from build123d import *

# Parameters (mm, degrees)
F0_R     = 45
F0_R_2   = 3
F1_DEPTH = 25
F2_COUNT = 7


# Not quite as in the source:
# - a feature names something its author has since deleted; it is built from what else it names


with BuildPart() as f1:
    # F0 (on Front) → F1 (new body)
    with BuildSketch(Plane.XZ):
        Circle(F0_R)
        with BuildLine():
            ThreePointArc((40, 0), (-34.8753984239, -19.58842987), (20.8146707615, 34.1577148107))
            ThreePointArc((20.8146707615, 34.1577148107), (21.2557560399, 33.8849942478), (21.693268588, 33.6065781949))
            ThreePointArc((21.693268588, 33.6065781949), (35.126419854, 19.1346447116), (40, 0))
        make_face(mode=Mode.SUBTRACT)
        with BuildLine():
            ThreePointArc((20.8146707615, 34.1577148107), (4.7404997755, 21.9880977011), (-2.457993575, 3.1556722874))
            ThreePointArc((-2.457993575, 3.1556722874), (-0.7771850997, -3.9237715684), (3.4753115022, 1.9804570085))
            ThreePointArc((3.4753115022, 1.9804570085), (8.7719800119, 19.9895662469), (21.693268588, 33.6065781949))
            ThreePointArc((21.693268588, 33.6065781949), (21.2557560399, 33.8849942478), (20.8146707615, 34.1577148107))
        make_face()
        Circle(F0_R_2, mode=Mode.SUBTRACT)
    extrude(amount=F1_DEPTH)

    # F2: F1 ×7 about axis
    f2_axis = Axis((0, -25, 0), (0, -1, 0))


with BuildPart() as f1_1:
    add(f1.part)
    for i in range(1, F2_COUNT):
        add(f1.part.rotate(f2_axis, i * 360 / F2_COUNT))


solid = f1_1.part
Model file for the job. Use its own axes, mm. Give positions to 0.01 mm unless a question says otherwise; leave off trailing zeros. Order: outer loops, then holes, each group sorted by start corner. A loop starts at its lowest first (then second) coordinate and runs counter-clockwise, first axis right, second up. Notation, with made-up numbers: (-31.5, -8.5) - (19.5, -8.5) arc R19 cw to (19.5, 6.5) - close; hole circle Ø1 at (-32.5, 24.5). An arc over 180 degrees is marked (long way). Return JSON: item names as keys, results as strings.
1) Pull direction X, two halves, no side cores. Call faces 1 (the flat face through (-4, 0, -3)), 2 (the cylindrical face through (21.6, -12.325, -11.034)): pulls with the +X half, pulls with the -X half, needs draft (parallel to the pull), parting line crosses it, or undercut.
Geometry says:
{"face 1": "needs draft", "face 2": "undercut"}
2) Cut at C-C, the plane x = 11. Give the cut face in (y, z), plus the area to 3 significant figures.
Geometry says:
{"outline": "(-25, -43.63) - (0, -43.63) - (0, -38.46) - (-25, -38.46) - close; (-25, -8.09) - (0, -8.09) - (0, -1.61) - (-25, -1.61) - close; (-25, 2.68) - (0, 2.68) - (0, 8.56) - (-25, 8.56) - close; (-25, 23.44) - (0, 23.44) - (0, 28.48) - (-25, 28.48) - close; (-25, 38.46) - (0, 38.46) - (0, 43.63) - (-25, 43.63) - close", "area": "694 mm²"}
3) Flat gauge pins, fed straight in: P1, Ø3, axis at y = -22, z = 18, coming from the +X side; P2, Ø6, axis at x = -18.5, y = -20, coming from the -Z side; P3, Ø1, axis at y = -19.5, z = 25.5, coming from the -X side. Where does each tip first touch, or does it go through?
Geometry says:
{"P1": "x = 41.87", "P2": "z = -42.25", "P3": "x = -37.42"}
4) Cut at A-A, the plane y = -2.25. Count the separate pieces of the cut face and the enclosed holes in it, plus the area to 3 significant figures.
Geometry says:
{"separate pieces": "1", "enclosed holes": "8", "area": "2,420 mm²"}
5) Probe line 1 (X direction, y = -12, z = 0); line 2 (X direction, y = -7, z = 30); line 3 (Z direction, x = 14, y = -18.5). List the from-to ranges inside material, lowest first. Write a range as from..to.
Geometry says:
{"line 1": "-45..-40, -23.09..-3, 3..7.94, 40..45", "line 2": "-33.54..-26.46, -15.25..-12.74, 13.02..16.94, 26.46..33.54", "line 3": "-42.77..-37.47, -10.08..-3.58, 3.85..9.3, 27.11..30.66, 37.47..42.77"}
6) Cut at B-B, the plane z = 29.5. Give the cut face in (x, y), plus the area to 3 significant figures.
Geometry says:
{"outline": "(-33.98, -25) - (-27.01, -25) - (-27.01, 0) - (-33.98, 0) - close; (-15.29, -25) - (-12.69, -25) - (-12.69, 0) - (-15.29, 0) - close; (12.32, -25) - (16.39, -25) - (16.39, 0) - (12.32, 0) - close; (27.01, -25) - (33.98, -25) - (33.98, 0) - (27.01, 0) - close", "area": "515 mm²"}
7) Cut at D-D, the plane z = 11.5. Give the cut face in (x, y).
Geometry says:
{"outline": "(-43.51, -25) - (-38.31, -25) - (-38.31, 0) - (-43.51, 0) - close; (-37.09, -25) - (-35.17, -25) - (-35.17, 0) - (-37.09, 0) - close; (-12.15, -25) - (-6.03, -25) - (-6.03, 0) - (-12.15, 0) - close; (-0.74, -25) - (5.11, -25) - (5.11, 0) - (-0.74, 0) - close; (38.31, -25) - (43.51, -25) - (43.51, 0) - (38.31, 0) - close"}
